For this review, take the finished solid that the model builds, in its own axes (mm). A direction names the side the tool comes from. Round coordinates to 2 decimals unless told otherwise and drop trailing zeros. Loops run counter-clockwise (first coordinate to the right, second up) from the corner with the lowest first, then second, coordinate; pieces in that order, holes last.
1) Tool access review of faces 5 (the flat face through (0, 8, -3)), 6 (the flat face through (0, -13, -3.525)), 7 (the cylindrical face through (2.588, 11.654, -0.786)): name each direction out of +Z, -Z, +X, -X, +Y, -Y from which nothing blocks a thin tool from reaching the whole face with its end or side.
2) Take a section at C-C (z = 2). State the section outline as (x, y) points, then the cut area to 3 significant figures.
3) Take a section at B-B (y = 0). State the section outline as (x, z) points.
4) Wall thickness on L1, parallel to X at y = -0.5, z = 3.25; L2, parallel to Y at x = 0, z = 1.95; L3, parallel to Z at x = -3.5, y = 10.5: over which ranges is each line inside the solid? List them lowest first.
5) Insertion check: pin 1 (4 mm diameter, centred on y = 12, z = 3, fed in from +X); pin 2 (12 mm diameter, centred on x = -1.5, y = -2, fed in from +Z); pin 3 (1.3 mm diameter, centred on x = -16.57, y = 0, fed in from -Z); pin 4 (0.5 mm diameter, centred on x = 4.5, z = -3, fed in from +Y). Each pin has a flat end and moves straight along its axis. Give the tip position at first contact, or say it passes through.
6) Mouldability with a two-part tool opening along X and no side actions: class faces 1 (the flat face through (-5.1, 5.1, -1.525)), 2 (the flat face through (-4, 13, 5.785)), 3 (the cylindrical face through (-12.461, -3.924, 3.092)), 4 (the cylindrical face through (19.6, -0.86, 1.19)) as pulls with the +X half, pulls with the -X half, needs draft (parallel to the pull), parting line crosses it, or undercut.
7) Take a section at D-D (x = -16.57). State the section outline as (y, z) points.
8) Take a section at A-A (x = 0). State the section outline as (y, z) points.
```python
from build123d import *

# Parameters (mm, degrees)
SKETCH1_W          = 12.617819502
SKETCH1_H          = 2
SKETCH1_W_2        = 6.5532
SKETCH1_H_2        = 5.31
SKETCH2_R          = 1.0922
CUT_EXTRUDE1_DEPTH = 10.31
SKETCH3_W          = 45.123892984
SKETCH3_H          = 16
CUT_EXTRUDE2_DEPTH = 1
CHAMFER1_SIZE      = 0.5


with BuildPart() as part:
    # Sketch1 → Revolve1 (revolve)
    with BuildSketch(Plane(origin=(0, 0, 0), x_dir=(1, 0, 0), z_dir=(0, 1, 0))):
        with Locations((-13.308909751, 2.525473465)):
            Rectangle(SKETCH1_W, SKETCH1_H)
        Polygon((-11.938, 1.525473465), (-19.617819502, 1.525473465), (-19.617819502, -0.474526535), (-13.064619502, -0.474526535), (-11.938, -0.474526535), align=None)
        with Locations((-16.341219502, -3.129526535)):
            Rectangle(SKETCH1_W_2, SKETCH1_H_2)
    revolve(axis=Axis((0, 0, -25.411285606), (0, 0, 1)))

    # Sketch2 → Cut-Extrude1 (cut, through all)
    with BuildSketch(Plane(origin=(0, 0, -3.525473465), x_dir=(-1, 0, 0), z_dir=(0, 0, -1))):
        with Locations((16.57, 0)):
            Circle(SKETCH2_R)
        with Locations((-16.57, 0)):
            Circle(SKETCH2_R)
    extrude(amount=-CUT_EXTRUDE1_DEPTH, mode=Mode.SUBTRACT)

    # Sketch3 → Cut-Extrude2 (cut)
    with BuildSketch(Plane(origin=(0, 0, -3.525473465), x_dir=(-1, 0, 0), z_dir=(0, 0, -1))):
        Rectangle(SKETCH3_W, SKETCH3_H)
    extrude(amount=-CUT_EXTRUDE2_DEPTH, mode=Mode.SUBTRACT)

    # Chamfer1
    chamfer1_edges = [part.edges().sort_by_distance(p)[0] for p in [
        (11.938, 0, 0.474526535),
    ]]
    chamfer(chamfer1_edges, length=CHAMFER1_SIZE)


solid = part.part
```
Response:
1. face 5: -Z, +X, -X
1. face 6: -Z, +X, -X, +Y, -Y
1. face 7: +Z
2. outline: circle Ø39.24 at (0, 0); hole circle Ø2.18 at (-16.57, 0); hole circle Ø26.13 at (0, 0); hole circle Ø2.18 at (16.57, 0)
2. area: 665 mm2
3. outline: (-19.62, -2.53) - (-17.66, -2.53) - (-17.66, 5.78) - (-19.62, 5.78) - close; (-15.48, -2.53) - (-7, -2.53) - (-7, -1.53) - (-11.94, -1.53) - (-11.94, -0.03) - (-12.44, 0.47) - (-13.06, 0.47) - (-13.06, 5.78) - (-15.48, 5.78) - close; (7, -2.53) - (15.48, -2.53) - (15.48, 5.78) - (13.06, 5.78) - (13.06, 0.47) - (12.44, 0.47) - (11.94, -0.03) - (11.94, -1.53) - (7, -1.53) - close; (17.66, -2.53) - (19.62, -2.53) - (19.62, 5.78) - (17.66, 5.78) - close
4. L1: x = -19.61 to -17.54, -15.6 to -13.06, 13.06 to 15.6, 17.54 to 19.61
4. L2: y = -19.62 to -13.06, 13.06 to 19.62
4. L3: z = -3.53 to -1.53
5. pin 1: stops at x = 16.88
5. pin 2: stops at z = -1.53
5. pin 3: passes through
5. pin 4: stops at y = 19.15
6. face 1: undercut
6. face 2: needs draft
6. face 3: undercut
6. face 4: parting line crosses it
7. outline: (-10.5, -3.53) - (-8, -3.53) - (-8, -2.53) - (-1.09, -2.53) - (-1.09, 5.78) - (-10.5, 5.78) - close; (1.09, -2.53) - (8, -2.53) - (8, -3.53) - (10.5, -3.53) - (10.5, 5.78) - (1.09, 5.78) - close
8. outline: (-19.62, -3.53) - (-8, -3.53) - (-8, -2.53) - (-7, -2.53) - (-7, -1.53) - (-11.94, -1.53) - (-11.94, -0.03) - (-12.44, 0.47) - (-13.06, 0.47) - (-13.06, 5.78) - (-19.62, 5.78) - close; (7, -2.53) - (8, -2.53) - (8, -3.53) - (19.62, -3.53) - (19.62, 5.78) - (13.06, 5.78) - (13.06, 0.47) - (12.44, 0.47) - (11.94, -0.03) - (11.94, -1.53) - (7, -1.53) - close
